```python
from build123d import *

# Parameters (mm, degrees)
SKETCH1_R           = 41.275
SKETCH1_R_2         = 38.1
BOSS_EXTRUDE1_DEPTH = 609.6
SKETCH3_R           = 44.45
BOSS_EXTRUDE2_DEPTH = 25.4
SKETCH5_R           = 41.275
SKETCH5_R_2         = 38.1
BOSS_EXTRUDE4_DEPTH = 609.6
FILLET1_R           = 1.27


with BuildPart() as part:
    # Sketch1 → Boss-Extrude1 (new body)
    with BuildSketch(Plane.XY):
        with Locations(Location((0, 0, 0), (0, 0, 180))):
            Circle(SKETCH1_R)
        with Locations(Location((0, 0, 0), (0, 0, 180))):
            Circle(SKETCH1_R_2, mode=Mode.SUBTRACT)
    extrude(amount=BOSS_EXTRUDE1_DEPTH)

    # Sketch3 → Boss-Extrude2 (add)
    with BuildSketch(Plane.XY.offset(609.6)):
        Circle(SKETCH3_R)
    extrude(amount=BOSS_EXTRUDE2_DEPTH)

    # Sketch5 → Boss-Extrude4 (add)
    with BuildSketch(Plane.XY.offset(635)):
        with Locations(Location((0, 0, 0), (0, 0, 180))):
            Circle(SKETCH5_R)
        with Locations(Location((0, 0, 0), (0, 0, 180))):
            Circle(SKETCH5_R_2, mode=Mode.SUBTRACT)
    extrude(amount=BOSS_EXTRUDE4_DEPTH)

    # Fillet1
    fillet1_edges = [part.edges().sort_by_distance(p)[0] for p in [
        (-44.45, 0, 609.6),
        (-44.45, 0, 635),
        (41.275, 0, 635),
        (41.275, 0, 609.6),
    ]]
    fillet(fillet1_edges, radius=FILLET1_R)


solid = part.part
```
Check sheet for the modelled part. Datum: model origin and axes. Units: mm. A direction names the side the tool comes from. Give positions to 0.01 mm unless a question says otherwise; leave off trailing zeros. Write each loop counter-clockwise with the first axis right and the second up, starting at its lowest first coordinate (ties: lowest second). Pieces come first, ordered by that corner, then holes. Notation, with made-up numbers: (36, -20) - (55, -20) arc R11 ccw to (55, -7) - close; hole circle Ø4 at (-37, 51). An arc over 180 degrees is marked (long way). Answer as a JSON object with one key per item and string values. Group by question number.
1) Sectioned sample at A-A (y = 0). Record the cut outline in (x, z) (3 decimals).
2) Thickness scan on probe 1 along Y at (x, z) = (0, 767) (3 decimals); probe 2 along Z at (x, y) = (-23.5, -11); probe 3 along Y at (x, z) = (-11.5, 633). Record the ranges inside material, lowest first. Write a range as from..to.
3) Sectioned sample at C-C (z = 251). Record the cut outline in (x, y) (3 decimals), then the cut area to 3 significant figures.
4) Depth check by flat-ended pin: P1, Ø10, axis at y = -10, z = 794.5, coming from the -X side; P2, Ø1, axis at x = -12.5, y = 28, coming from the -Z side; P3, Ø3, axis at x = -15, z = 739, coming from the +Y side. Enter the tip coordinate at first touch or a pass-through.
5) Access from +Z, -Z, +X, -X, +Y, -Y to the whole of each face (thin tool, end or side, straight path). Record for faces 1 (the face through (31.8, -28.6, 635)), 2 (the face through (-12, 36.5, 1244.6)), 3 (the face through (-1, 1, 609.6)).
6) Release check for a two-part mould opening along X. For faces 4 (the face through (31.8, -28.6, 609.6)), 5 (the face through (8.259, 37.194, 935.533)), 6 (the face through (42.397, 13.352, 622.14)) record: pulls with the +X half, pulls with the -X half, needs draft (parallel to the pull), parting line crosses it, or undercut.
Geometry results:
{
 "1": {"outline": "(-44.45, 610.87) arc R1.27 ccw to (-43.18, 609.6) - (-42.545, 609.6) arc R1.27 cw to (-41.275, 608.33) - (-41.275, 0) - (-38.1, 0) - (-38.1, 609.6) - (38.1, 609.6) - (38.1, 0) - (41.275, 0) - (41.275, 608.33) arc R1.27 cw to (42.545, 609.6) - (43.18, 609.6) arc R1.27 ccw to (44.45, 610.87) - (44.45, 633.73) arc R1.27 ccw to (43.18, 635) - (42.545, 635) arc R1.27 cw to (41.275, 636.27) - (41.275, 1244.6) - (38.1, 1244.6) - (38.1, 635) - (-38.1, 635) - (-38.1, 1244.6) - (-41.275, 1244.6) - (-41.275, 636.27) arc R1.27 cw to (-42.545, 635) - (-43.18, 635) arc R1.27 ccw to (-44.45, 633.73) - close"},
 "2": {"probe 1": "y = -41.275..-38.1, 38.1..41.275", "probe 2": "z = 609.6..635", "probe 3": "y = -42.94..42.94"},
 "3": {"outline": "circle Ø82.55 at (0, 0); hole circle Ø76.2 at (0, 0)", "area": "792 mm^2"},
 "4": {"P1": "stops at x = -40.97", "P2": "stops at z = 609.6", "P3": "stops at y = 39"},
 "5": {"face 1": "+Z", "face 2": "+Z, +X, -X, +Y, -Y", "face 3": "-Z"},
 "6": {"face 4": "needs draft", "face 5": "undercut", "face 6": "parting line crosses it"}
}
